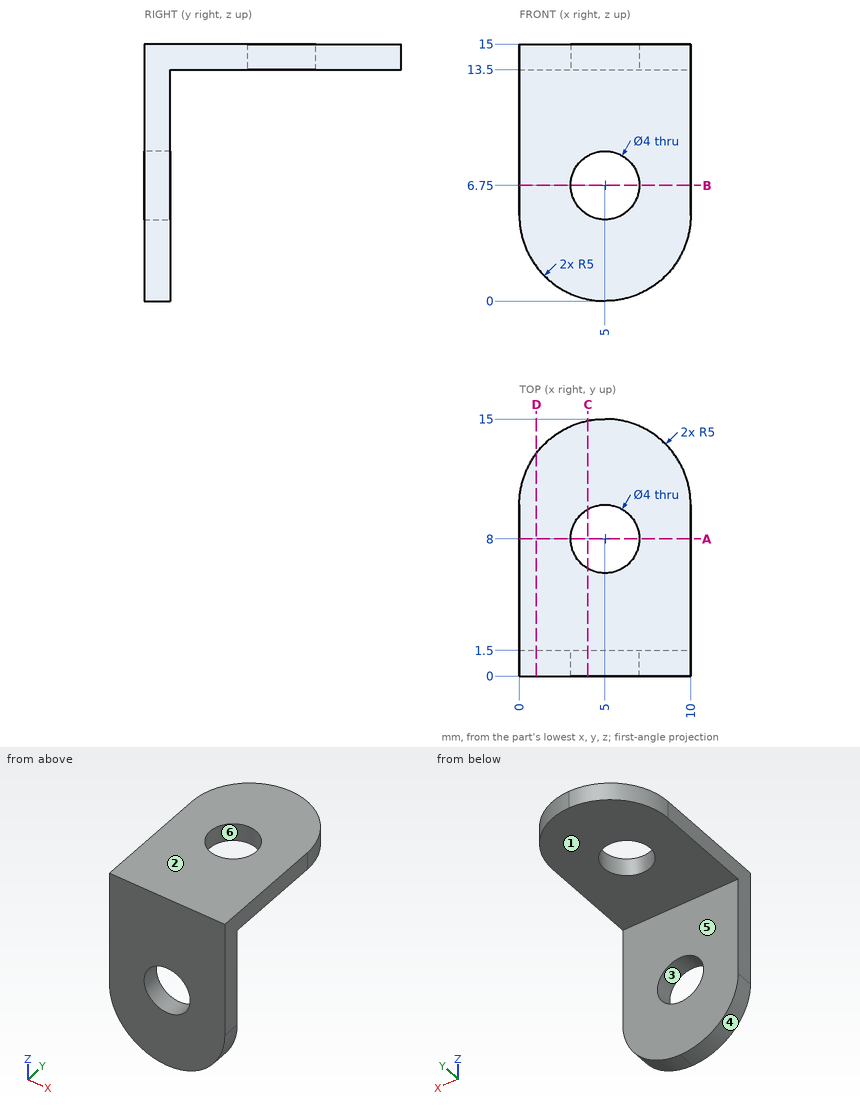
Here's the drawing with two shaded views (mm, measured from the low corner). I have some questions. A direction names the side the tool comes from. Give positions to 0.01 mm unless a question says otherwise; leave off trailing zeros. Loops run counter-clockwise (first coordinate to the right, second up) from the corner with the lowest first, then second, coordinate; pieces in that order, holes last. Notation, with made-up numbers: (33, 19.5) - (45, 19.5) arc R22 cw to (45, 55.5) - close; hole circle Ø2 at (42.25, -5). An arc over 180 degrees is marked (long way). Answer in a Markdown table with one row per item. Add a question column.
Q1. If we section it at B-B (z = 6.75): List the corners of the cut face in (x, y) for me, plus the area to 3 significant figures.
Q2. If we section it at C-C (x = 4): List the corners of the cut face in (y, z) for me.
Q3. For pin 1 (2.5 mm diameter, centred on x = 5, y = 8, fed in from -Z); pin 2 (5 mm diameter, centred on x = 1.5, y = 12.5, fed in from -Z); pin 3 (3 mm diameter, centred on x = 5.5, z = 2, fed in from +Y), each with a flat end and sliding along its axis, tell me the tip position at first contact or that it passes through.
Q4. Please list where these lines run through material, in increasing order: L1, parallel to X at y = 8, z = 14.75; L2, parallel to Y at x = 6, z = 12.5; L3, parallel to Z at x = 1.75, y = 13.75. Write a range as from..to.
Q5. We'd pull the mould along X, two halves only. Please class the marked faces 3, 4, 5 and 6: +X half, -X half, draft (parallel to the pull), parting line (faces both ways), or undercut.
Q6. Which directions (+Z, -Z, +X, -X, +Y, -Y) give clear straight access to the entire face, cutting with the end or side of a thin tool? Please do the marked faces 1 and 2.
Q7. If we section it at D-D (x = 1): List the corners of the cut face in (y, z) for me.
Q8. If we section it at A-A (y = 8): List the corners of the cut face in (x, z) for me, plus the area to 3 significant figures.
The answers:
| question | item | result |
|---|---|---|
| 1 | outline | (0, 0) - (3, 0) - (3, 1.5) - (0, 1.5) - close; (7, 0) - (10, 0) - (10, 1.5) - (7, 1.5) - close |
| 1 | area | 9.00 mm^2 |
| 2 | outline | (0, 0.1) - (1.5, 0.1) - (1.5, 5.02) - (0, 5.02) - close; (0, 8.48) - (1.5, 8.48) - (1.5, 13.5) - (6.27, 13.5) - (6.27, 15) - (0, 15) - close; (9.73, 13.5) - (14.9, 13.5) - (14.9, 15) - (9.73, 15) - close |
| 3 | pin 1 | passes through |
| 3 | pin 2 | stops at z = 13.5 |
| 3 | pin 3 | stops at y = 1.5 |
| 4 | L1 | x = 0..3, 7..10 |
| 4 | L2 | y = 0..1.5 |
| 4 | L3 | z = 13.5..15 |
| 5 | face 3 | undercut |
| 5 | face 4 | -X half |
| 5 | face 5 | draft |
| 5 | face 6 | undercut |
| 6 | face 1 | -Z, +X, -X, +Y |
| 6 | face 2 | +Z, +X, -X, +Y, -Y |
| 7 | outline | (0, 2) - (1.5, 2) - (1.5, 13.5) - (13, 13.5) - (13, 15) - (0, 15) - close |
| 8 | outline | (0, 13.5) - (3, 13.5) - (3, 15) - (0, 15) - close; (7, 13.5) - (10, 13.5) - (10, 15) - (7, 15) - close |
| 8 | area | 9.00 mm^2 |
